Part model, mm, in its own coordinate system. Face numbers are marked on the shaded views. A direction names the side the tool comes from. Coordinates: 2 decimals unless noted, no trailing zeros. Loops run counter-clockwise (first coordinate to the right, second up) from the corner with the lowest first, then second, coordinate; pieces in that order, holes last. Notation, with made-up numbers: (82.25, 50.5) - (108.25, 50.5) arc R24 ccw to (108.25, 80.5) - close; hole circle Ø4 at (-1, 0). An arc over 180 degrees is marked (long way). Answer as CSV lines item,"result".
from build123d import *

# Parameters (mm, degrees)
SKETCH1_R           = 50.8
BOSS_EXTRUDE1_DEPTH = 38.1
SKETCH1_3_R         = 50.8
BOSS_EXTRUDE2_DEPTH = 6.35
SKETCH2_R           = 38.1
BOSS_EXTRUDE3_DEPTH = 107.95
SKETCH3_R           = 12.7
CUT_EXTRUDE1_DEPTH  = 153.4
CUT_EXTRUDE2_DEPTH  = 38.1


with BuildPart() as part:
    # Sketch1 → Boss-Extrude1 (new body)
    with BuildSketch(Plane(origin=(0, 0, 0), x_dir=(0, 0, -1), z_dir=(1, 0, 0))):
        with BuildLine():
            ThreePointArc((-50.8, 4.8e-08), (-43.994090395, 25.400000202), (-25.399999637, 43.994090722))
            Line((-25.399999637, 43.994090722), (-50.8, 29.329393675))
            Line((-50.8, 29.329393675), (-50.8, 4.8e-08))
        make_face()
        with BuildLine():
            ThreePointArc((-25.399999637, 43.994090722), (3.52e-07, 50.8), (25.400000247, 43.99409037))
            Line((25.400000247, 43.99409037), (0, 58.65878735))
            Line((0, 58.65878735), (-25.399999637, 43.994090722))
        make_face()
        Circle(SKETCH1_R)
        with BuildLine():
            Line((50.8, 0), (50.8, 29.329393675))
            Line((50.8, 29.329393675), (25.400000247, 43.99409037))
            ThreePointArc((25.400000247, 43.99409037), (43.994090583, 25.399999877), (50.8, 0))
        make_face()
        with BuildLine():
            Line((50.8, -29.329393675), (50.8, 0))
            ThreePointArc((50.8, 0), (43.994090529, -25.39999997), (25.400000059, -43.994090478))
            Line((25.400000059, -43.994090478), (50.8, -29.329393675))
        make_face()
        with BuildLine():
            Line((0, -58.65878735), (25.400000059, -43.994090478))
            ThreePointArc((25.400000059, -43.994090478), (-2.2e-07, -50.8), (-25.400000441, -43.994090258))
            Line((-25.400000441, -43.994090258), (0, -58.65878735))
        make_face()
        with BuildLine():
            ThreePointArc((-25.400000441, -43.994090258), (-43.994090651, -25.399999759), (-50.8, 4.8e-08))
            Line((-50.8, 4.8e-08), (-50.8, -29.329393675))
            Line((-50.8, -29.329393675), (-25.400000441, -43.994090258))
        make_face()
    extrude(amount=-BOSS_EXTRUDE1_DEPTH)

    # Sketch1_3 → Boss-Extrude2 (add)
    with BuildSketch(Plane(origin=(0, 0, 0), x_dir=(0, 0, -1), z_dir=(1, 0, 0))):
        Circle(SKETCH1_3_R)
    extrude(amount=BOSS_EXTRUDE2_DEPTH)

    # Sketch2 → Boss-Extrude3 (add)
    with BuildSketch(Plane(origin=(6.35, 0, 0), x_dir=(0, 0, -1), z_dir=(1, 0, 0))):
        Circle(SKETCH2_R)
    extrude(amount=BOSS_EXTRUDE3_DEPTH)

    # Sketch3 → Cut-Extrude1 (cut, through all)
    with BuildSketch(Plane(origin=(114.3, 0, 0), x_dir=(0, 0, -1), z_dir=(1, 0, 0))):
        Circle(SKETCH3_R)
    extrude(amount=-CUT_EXTRUDE1_DEPTH, mode=Mode.SUBTRACT)

    # Sketch3_3 → Cut-Extrude2 (cut)
    with BuildSketch(Plane(origin=(114.3, 0, 0), x_dir=(0, 0, -1), z_dir=(1, 0, 0))):
        with BuildLine():
            Line((-25.4, -28.398063314), (-25.4, 28.398063314))
            ThreePointArc((-25.4, 28.398063314), (-38.1, 0), (-25.4, -28.398063314))
        make_face()
        with BuildLine():
            ThreePointArc((38.1, 0), (34.780382402, 15.554259867), (25.4, 28.398063314))
            Line((25.4, 28.398063314), (25.4, -28.398063314))
            ThreePointArc((25.4, -28.398063314), (34.780382402, -15.554259867), (38.1, 0))
        make_face()
    extrude(amount=-CUT_EXTRUDE2_DEPTH, mode=Mode.SUBTRACT)


solid = part.part
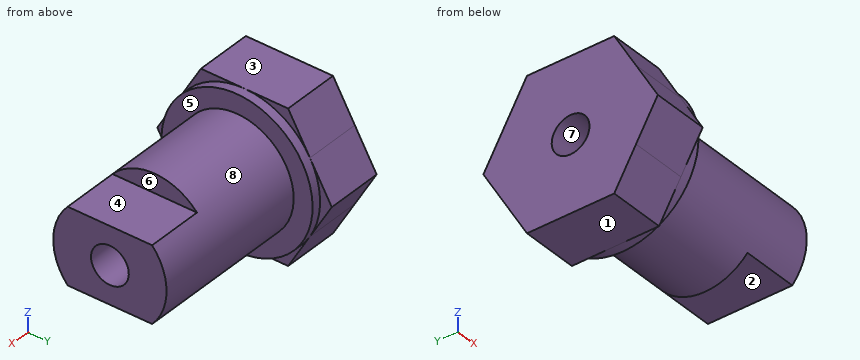
Q1. Flat gauge pins, fed straight in: pin 1 (4 mm diameter, centred on x = 46.5, z = -8, fed in from +Y); pin 2 (6.5 mm diameter, centred on y = 4, z = 32, fed in from +X); pin 3 (12 mm diameter, centred on x = 35.5, z = 37, fed in from -Y); pin 4 (15 mm diameter, centred on y = 0, z = 0, fed in from -X). Where does each tip first touch, or does it go through?
Results:
pin 1,"stops at y = 37.62"
pin 2,"stops at x = 76.2"
pin 3,"stops at y = -22.15"
pin 4,"passes through"
Q2. Saw through at D-D (y = 17.5). Give the cut face in (x, z), then the cut area to 3 significant figures.
Results:
outline,"(-38.1, -50.8) - (0, -50.8) - (0, -47.69) - (6.35, -47.69) - (6.35, -33.84) - (76.2, -33.84) - (76.2, -25.4) - (114.3, -25.4) - (114.3, 25.4) - (76.2, 25.4) - (76.2, 33.84) - (6.35, 33.84) - (6.35, 47.69) - (0, 47.69) - (0, 50.8) - (-38.1, 50.8) - close"
area,"11,100 mm^2"
Q3. Saw through at B-B (x = 98.5). Give the cut face in (y, z).
Results:
outline,"(-28.4, -25.4) - (28.4, -25.4) arc R38.1 ccw to (28.4, 25.4) - (-28.4, 25.4) arc R38.1 ccw to start; hole circle Ø25.4 at (0, 0)"
Q4. Saw through at A-A (z = -10). Give the cut face in (x, y).
Results:
outline,"(-38.1, -52.89) - (0, -52.89) - (0, -49.81) - (6.35, -49.81) - (6.35, -36.76) - (114.3, -36.76) - (114.3, -7.83) - (-38.1, -7.83) - close; (-38.1, 7.83) - (114.3, 7.83) - (114.3, 36.76) - (6.35, 36.76) - (6.35, 49.81) - (0, 49.81) - (0, 52.89) - (-38.1, 52.89) - close"
Q5. Two-plate mould, pull along Y, no slides. Class the marked faces 6, 7 and 8: released by +Y, released by -Y, zero draft, split by the parting line, or undercut.
Results:
face 6,"zero draft"
face 7,"undercut"
face 8,"split by the parting line"
Q6. Wall check: L1, parallel to Y at x = 47, z = 0; L2, parallel to X at y = -9.5, z = -27; L3, parallel to X at y = 25, z = 33.5. Give the ranges that are in metal, low to high.
Results:
L1,"y = -38.1 to -12.7, 12.7 to 38.1"
L2,"x = -38.1 to 76.2"
L3,"x = -38.1 to 6.35"
Q7. Which spindle directions (+Z, -Z, +X, -X, +Y, -Y) get a long thin tool onto all of the face, cutting with end or side? Do the marked faces 1, 2, 3, 4 and 5. Say none if no direction does.
Results:
face 1,"-Z, +X, -X, +Y, -Y"
face 2,"-Z, +X, +Y, -Y"
face 3,"+Z, +X, -X, +Y, -Y"
face 4,"+Z, +X, +Y, -Y"
face 5,"+X"
